Model file for the job. Use its own axes, mm. Face numbers are marked on the shaded views. A direction names the side the tool comes from. Round coordinates to 2 decimals unless told otherwise and drop trailing zeros. Write each loop counter-clockwise with the first axis right and the second up, starting at its lowest first coordinate (ties: lowest second). Pieces come first, ordered by that corner, then holes.
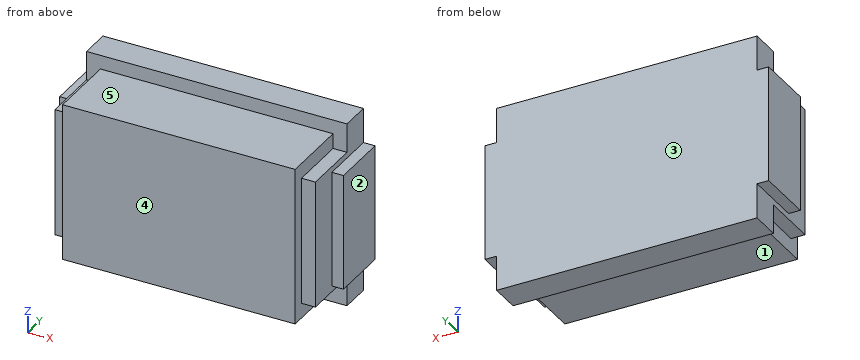
Autodesk Inventor part; units mm, degrees
ref_plane "YZ Plane" through (0, 0, 0) normal (1, 0, 0) x (0, 1, 0)
ref_plane "XZ Plane" through (0, 0, 0) normal (0, 1, 0) x (-1, 0, 0)
ref_plane "XY Plane" through (0, 0, 0) normal (0, 0, 1) x (1, 0, 0)
sketch "Esquisse1" plane through (0, 0, 0) normal (0, 1, 0) x (-1, 0, 0)
  line L0 (-50, 34) -> (50, 34)
  line L1 (50, 34) -> (50, -34)
  line L2 (50, -34) -> (-50, -34)
  line L3 (-50, -34) -> (-50, 34)
  point P0 (0, 0)
  dimension "d0" = 100
  dimension "d1" = 68
  dimension "d2" = 34
  dimension "d3" = 50
extrude "Extrusion1" add sketch "Esquisse1" along normal blind 30
sketch "Esquisse2" plane through (0, 30, 0) normal (0, 1, 0) x (1, 0, 0)
  line L0 (-56, 40) -> (56, 40)
  line L1 (56, 40) -> (56, -40)
  line L2 (56, -40) -> (-56, -40)
  line L3 (-56, -40) -> (-56, 40)
  point P0 (0, 0)
  dimension "d6" = 112
  dimension "d7" = 80
  dimension "d8" = 40
  dimension "d9" = 56
extrude "Extrusion2" add sketch "Esquisse2" along normal blind 13
sketch "Esquisse3" plane through (50, 0, 34) normal (1, 0, 0) x (0, 0, -1)
  line L0 (0, 30) -> (68, 30)
  line L1 (6.5, 30) -> (61.5, 30)
  line L2 (61.5, 30) -> (61.5, 5)
  line L3 (61.5, 5) -> (6.5, 5)
  line L4 (6.5, 5) -> (6.5, 30)
  point P0 (34, 0)
  dimension "d12" = 25
  dimension "d13" = 55
  dimension "d14" = 27.5
extrude "Extrusion3" add sketch "Esquisse3" along normal up to surface (6 mm away)
sketch "Esquisse4" plane through (56, 30, -40) normal (1, 0, 0) x (0, 0, -1)
  line L0 (-80, 13) -> (0, 13)
  line L1 (-65, 13) -> (-15, 13)
  line L2 (-15, 13) -> (-15, -12)
  line L3 (-15, -12) -> (-65, -12)
  line L4 (-65, -12) -> (-65, 13)
  point P0 (-40, -30)
  dimension "d17" = 50
  dimension "d18" = 25
  dimension "d19" = 25
extrude "Extrusion4" add sketch "Esquisse4" along normal blind 5
mirror "Symétrie1" about plane through (0, 0, 0) normal (1, 0, 0) of "Extrusion4", "Extrusion3"
properties part number "leroy_merlin_boite"
1) Cut at C-C on z = 30. List the corners of the cut face in (x, y).
2) Which spindle directions (+Z, -Z, +X, -X, +Y, -Y) get a long thin tool onto all of the face, cutting with end or side? Do the marked faces 1 and 2. Say none if no direction does.
3) Cut at B-B on y = 12.5. List the corners of the cut face in (x, z).
4) Cut at A-A on x = -53. List the corners of the cut face in (y, z), and give its area (4 significant figures).
5) Flat gauge pins, fed straight in: pin 1 Ø5.5 at (x, z) = (59, 1) entering from -Y; pin 2 Ø6.5 at (x, z) = (51.5, -11.5) entering from -Y; pin 3 Ø2 at (x, y) = (-2, 19.5) entering from +Z; pin 4 Ø9 at (y, z) = (10.5, -2.5) entering from -X. Where does each tip first touch, or does it go through?
6) Pull direction Y, two halves, no side cores. Call the marked faces 3, 4 and 5: released by +Y, released by -Y, zero draft, split by the parting line, or undercut.
7) Cut at D-D on y = 28.5. List the corners of the cut face in (x, z).
8) Wall check: probe 1 along X at (y, z) = (15.5, 33); probe 2 along Z at (x, y) = (26, 27); probe 3 along Y at (x, z) = (-54, 30). Give the ranges that are in metal, low to high.
Result sheet:
1. outline: (-56, 30) - (-50, 30) - (-50, 0) - (50, 0) - (50, 30) - (56, 30) - (56, 43) - (-56, 43) - close
2. face 1: -Z, +X, -X, -Y
2. face 2: +Z, -Z, +X, +Y, -Y
3. outline: (-56, -27.5) - (-50, -27.5) - (-50, -34) - (50, -34) - (50, -27.5) - (56, -27.5) - (56, 27.5) - (50, 27.5) - (50, 34) - (-50, 34) - (-50, 27.5) - (-56, 27.5) - close
4. outline: (5, -27.5) - (30, -27.5) - (30, -40) - (43, -40) - (43, 40) - (30, 40) - (30, 27.5) - (5, 27.5) - close
4. area: 2,415 mm2
5. pin 1: stops at y = 18
5. pin 2: stops at y = 0
5. pin 3: stops at z = 34
5. pin 4: stops at x = -56
6. face 3: released by +Y
6. face 4: released by -Y
6. face 5: zero draft
7. outline: (-61, -25) - (-56, -25) - (-56, -27.5) - (-50, -27.5) - (-50, -34) - (50, -34) - (50, -27.5) - (56, -27.5) - (56, -25) - (61, -25) - (61, 25) - (56, 25) - (56, 27.5) - (50, 27.5) - (50, 34) - (-50, 34) - (-50, 27.5) - (-56, 27.5) - (-56, 25) - (-61, 25) - close
8. probe 1: x = -50 to 50
8. probe 2: z = -34 to 34
8. probe 3: y = 30 to 43
